For this review, take the finished solid that the model builds, in its own axes (mm). Face numbers are marked on the shaded views. A direction names the side the tool comes from. Coordinates: 2 decimals unless noted, no trailing zeros. Loops run counter-clockwise (first coordinate to the right, second up) from the corner with the lowest first, then second, coordinate; pieces in that order, holes last.
1. Take a section at A-A, the plane z = 5. State the section outline as (x, y) points, then the cut area to 3 significant figures.
2. Take a section at D-D, the plane z = 8.25. State the section outline as (x, y) points, then the cut area to 3 significant figures.
3. To check wall thickness, follow probe 1 along X at (y, z) = (-2.75, 3.5); probe 2 along Y at (x, z) = (2.25, 5.5); probe 3 along X at (y, z) = (-4, 2.75). State the ranges of each line that lie inside material, in increasing order.
4. Clearance check with flat-ended pins moving along their axes: P1, Ø1, axis at y = -3, z = 2, coming from the +X side; P2, Ø5, axis at x = 5.5, z = 2.5, coming from the -Y side; P3, Ø2, axis at x = 4.5, z = 5, coming from the +Y side. State where each tip first meets the part, or that it passes through.
5. Take a section at B-B, the plane x = 8.25. State the section outline as (y, z) points, then the cut area to 3 significant figures.
6. Machinability: for the marked faces 1, 2, 3 and 4, which of the approach directions +Z, -Z, +X, -X, +Y, -Y give a long, thin tool a straight path to every point of the face, cutting with its end or side? Answer none if there is none.
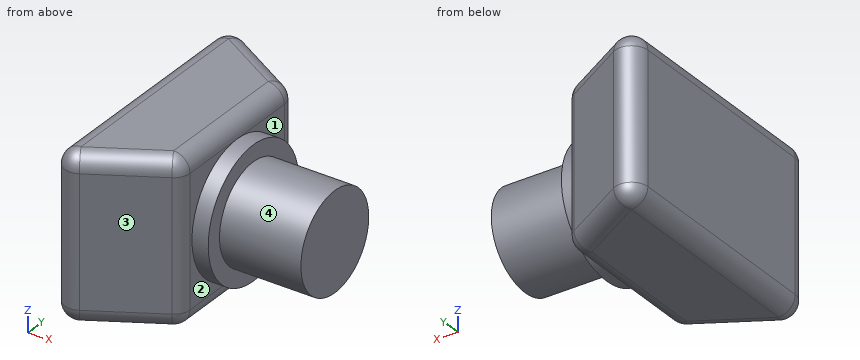
```python
from build123d import *

# Parameters (mm, degrees)
Y_KSEKLIK_EKSTR_ZYON1_DEPTH = 10
RADYUS1_R                   = 1
RADYUS2_R                   = 1
IZIM2_R                     = 4
Y_KSEKLIK_EKSTR_ZYON2_DEPTH = 1
IZIM3_R                     = 3
Y_KSEKLIK_EKSTR_ZYON3_DEPTH = 5


with BuildPart() as part:
    # Çizim1 → Yükseklik-Ekstrüzyon1 (new body)
    with BuildSketch(Plane.XY):
        Polygon((0, -8.25), (0, 8.25), (6.062177826, 4.75), (6.062177826, -4.75), align=None)
    extrude(amount=Y_KSEKLIK_EKSTR_ZYON1_DEPTH)

    # Radyus1
    radyus1_edges = [part.edges().sort_by_distance(p)[0] for p in [
        (0, -8.25, 5),
        (0, 8.25, 5),
        (6.062177826, 4.75, 5),
        (6.062177826, -4.75, 5),
    ]]
    fillet(radyus1_edges, radius=RADYUS1_R)

    # Radyus2
    radyus2_edges = [part.edges().sort_by_distance(p)[0] for p in [
        (3.531088913, -6.211324865, 0),
        (3.531088913, -6.211324865, 10),
        (0, 0, 0),
        (3.531088913, 6.211324865, 0),
        (6.062177826, 0, 0),
        (0.5, 7.383974596, 0),
        (5.92820323, 4.672649731, 0),
        (5.92820323, -4.672649731, 0),
        (0.5, -7.383974596, 0),
        (0, 0, 10),
        (6.062177826, 0, 10),
        (3.531088913, 6.211324865, 10),
        (0.5, 7.383974596, 10),
        (5.92820323, 4.672649731, 10),
        (5.92820323, -4.672649731, 10),
        (0.5, -7.383974596, 10),
    ]]
    fillet(radyus2_edges, radius=RADYUS2_R)

    # Çizim2 → Yükseklik-Ekstrüzyon2 (add)
    with BuildSketch(Plane(origin=(6.062177826, 0, 0), x_dir=(0, 0, -1), z_dir=(1, 0, 0))):
        with Locations((-5, 0)):
            Circle(IZIM2_R)
    extrude(amount=Y_KSEKLIK_EKSTR_ZYON2_DEPTH)

    # Çizim3 → Yükseklik-Ekstrüzyon3 (add)
    with BuildSketch(Plane(origin=(7.062177826, 0, 0), x_dir=(0, 0, -1), z_dir=(1, 0, 0))):
        with Locations(Location((-5, 0, 0), (0, 0, 90))):
            Circle(IZIM3_R)
    extrude(amount=Y_KSEKLIK_EKSTR_ZYON3_DEPTH)


solid = part.part
```
Results list:
1. outline: (0, -6.52) arc R1 ccw to (1.5, -7.38) - (5.56, -5.04) arc R1 ccw to (6.06, -4.17) - (6.06, -4) - (7.06, -4) - (7.06, -3) - (12.06, -3) - (12.06, 3) - (7.06, 3) - (7.06, 4) - (6.06, 4) - (6.06, 4.17) arc R1 ccw to (5.56, 5.04) - (1.5, 7.38) arc R1 ccw to (0, 6.52) - close
1. area: 115 mm2
2. outline: (0, -6.52) arc R1 ccw to (1.5, -7.38) - (5.56, -5.04) arc R1 ccw to (6.06, -4.17) - (6.06, -2.33) - (7.06, -2.33) - (7.06, 2.33) - (6.06, 2.33) - (6.06, 4.17) arc R1 ccw to (5.56, 5.04) - (1.5, 7.38) arc R1 ccw to (0, 6.52) - close
2. area: 82.0 mm2
3. probe 1: x = 0 to 7.06
3. probe 2: y = -6.95 to 6.95
3. probe 3: x = 0 to 6.06
4. P1: stops at x = 7.06
4. P2: stops at y = -6.52
4. P3: stops at y = 6.23
5. outline: circle Ø6 at (0, 5)
5. area: 28.3 mm2
6. face 1: +X, +Y
6. face 2: +X, -Y
6. face 3: +Z, -Z, +X, -Y
6. face 4: +X
